Can you work these out from the model? Positions are in its coordinate system, mm. Face numbers are marked on the shaded views. Give positions to 0.01 mm unless a question says otherwise; leave off trailing zeros. Write each loop counter-clockwise with the first axis right and the second up, starting at its lowest first coordinate (ties: lowest second). Pieces come first, ordered by that corner, then holes. Notation, with made-up numbers: (69.25, 82) -> (81.25, 82) arc R14 cw to (81.25, 89) -> close; hole circle Ø5 at (55, 82.25). An arc over 180 degrees is marked (long way). Answer as CSV lines item,"result". Start each with the question number.
1. If we section it at A-A on y = 14: Count the separate pieces of the cut face and the enclosed holes in it, plus the area to 3 significant figures.
2. I'm going to push flat-ended pins straight in: P1, Ø3, axis at x = 28.5, z = -5.5, coming from the -Y side; P2, Ø2, axis at x = 42.5, y = 13.5, coming from the -Z side; P3, Ø3, axis at y = 13.5, z = -19.5, coming from the +X side; P4, Ø3, axis at x = 72.5, y = 14.5, coming from the +Z side. Where does each tip first touch, or does it pass through?
3. If we mould it in two halves opening along X, with no side actions, what happens to the marked faces 1 and 2? For each: pulls with the +X half, pulls with the -X half, needs draft (parallel to the pull), parting line crosses it, or undercut.
4. I need wall thicknesses on line 1 (Z direction, x = 28.5, y = 3.5); line 2 (Z direction, x = 28.5, y = 2.1) (3 decimals); line 3 (X direction, y = 3.4, z = -5.5). Which ranges of each line are inside material? Lowest first, please. Write a range as [from, to].
5. If we section it at B-B on x = 168.5: Write out the boundary of the cut face in (y, z), plus the area to 3 significant figures.
```python
from build123d import *

# Parameters (mm, degrees)
SKETCH1_W                = 240
SKETCH1_H                = 35
SKETCH1_W_2              = 12.7
SKETCH1_H_2              = 12.7
BOSS_EXTRUDE1_DEPTH      = 4
SKETCH2_W                = 12.7
SKETCH2_H                = 12.7
BOSS_EXTRUDE2_DEPTH      = 13
BOSS_EXTRUDE2_DEPTH_BACK = 4
CHAMFER1_SIZE            = 0.2
CHAMFER1_SIZE2           = 8
SKETCH3_R                = 1.725
CUT_EXTRUDE1_DEPTH       = 5
SKETCH4_R                = 3
CUT_EXTRUDE2_DEPTH       = 1
FILLET1_R                = 1


with BuildPart() as part:
    # Sketch1 → Boss-Extrude1 (new body)
    with BuildSketch(Plane(origin=(0, 0, 0), x_dir=(1, 0, 0), z_dir=(0, 1, 0))):
        with Locations((120, 17.5)):
            Rectangle(SKETCH1_W, SKETCH1_H)
        with Locations((13.25, 17.5)):
            Rectangle(SKETCH1_W_2, SKETCH1_H_2, mode=Mode.SUBTRACT)
        with Locations((43.75, 17.5)):
            Rectangle(SKETCH1_W_2, SKETCH1_H_2, mode=Mode.SUBTRACT)
        with Locations((74.25, 17.5)):
            Rectangle(SKETCH1_W_2, SKETCH1_H_2, mode=Mode.SUBTRACT)
        with Locations((104.75, 17.5)):
            Rectangle(SKETCH1_W_2, SKETCH1_H_2, mode=Mode.SUBTRACT)
        with Locations((135.25, 17.5)):
            Rectangle(SKETCH1_W_2, SKETCH1_H_2, mode=Mode.SUBTRACT)
        with Locations((165.75, 17.5)):
            Rectangle(SKETCH1_W_2, SKETCH1_H_2, mode=Mode.SUBTRACT)
        with Locations((196.25, 17.5)):
            Rectangle(SKETCH1_W_2, SKETCH1_H_2, mode=Mode.SUBTRACT)
        with Locations((226.75, 17.5)):
            Rectangle(SKETCH1_W_2, SKETCH1_H_2, mode=Mode.SUBTRACT)
    extrude(amount=BOSS_EXTRUDE1_DEPTH)

    # Sketch2 → Boss-Extrude2 (add, two sides)
    with BuildSketch(Plane(origin=(0, 4, 0), x_dir=(1, 0, 0), z_dir=(0, 1, 0))) as boss_extrude2_sk:
        with Locations((13.25, 17.5)):
            Rectangle(SKETCH2_W, SKETCH2_H)
        with Locations((43.75, 17.5)):
            Rectangle(SKETCH2_W, SKETCH2_H)
        with Locations((74.25, 17.5)):
            Rectangle(SKETCH2_W, SKETCH2_H)
        with Locations((104.75, 17.5)):
            Rectangle(SKETCH2_W, SKETCH2_H)
        with Locations((135.25, 17.5)):
            Rectangle(SKETCH2_W, SKETCH2_H)
        with Locations((165.75, 17.5)):
            Rectangle(SKETCH2_W, SKETCH2_H)
        with Locations((196.25, 17.5)):
            Rectangle(SKETCH2_W, SKETCH2_H)
        with Locations((226.75, 17.5)):
            Rectangle(SKETCH2_W, SKETCH2_H)
    extrude(amount=BOSS_EXTRUDE2_DEPTH)
    extrude(boss_extrude2_sk.sketch, amount=-BOSS_EXTRUDE2_DEPTH_BACK)

    # Chamfer1
    chamfer1_edges = [part.edges().sort_by_distance(p)[0] for p in [
        (189.9, 4, -17.5),
        (196.25, 4, -11.15),
        (202.6, 4, -17.5),
        (196.25, 4, -23.85),
        (6.9, 4, -17.5),
        (13.25, 4, -11.15),
        (19.6, 4, -17.5),
        (13.25, 4, -23.85),
        (67.9, 4, -17.5),
        (74.25, 4, -11.15),
        (80.6, 4, -17.5),
        (74.25, 4, -23.85),
        (37.4, 4, -17.5),
        (43.75, 4, -11.15),
        (50.1, 4, -17.5),
        (43.75, 4, -23.85),
        (98.4, 4, -17.5),
        (104.75, 4, -11.15),
        (111.1, 4, -17.5),
        (104.75, 4, -23.85),
        (128.9, 4, -17.5),
        (135.25, 4, -11.15),
        (141.6, 4, -17.5),
        (135.25, 4, -23.85),
        (159.4, 4, -17.5),
        (165.75, 4, -11.15),
        (172.1, 4, -17.5),
        (165.75, 4, -23.85),
        (220.4, 4, -17.5),
        (226.75, 4, -11.15),
        (233.1, 4, -17.5),
        (226.75, 4, -23.85),
    ]]
    chamfer1_side = [part.faces().sort_by_distance(p)[0] for p in [
        (120, 4, -17.5),
    ]]
    chamfer(chamfer1_edges, length=CHAMFER1_SIZE, length2=CHAMFER1_SIZE2, reference=chamfer1_side[0])

    # Sketch3 → Cut-Extrude1 (cut, through all)
    with BuildSketch(Plane(origin=(0, 4, 0), x_dir=(1, 0, 0), z_dir=(0, 1, 0))):
        with Locations((28.5, 5.5)):
            Circle(SKETCH3_R)
        with Locations((28.5, 29.5)):
            Circle(SKETCH3_R)
        with Locations((211.6, 29.5)):
            Circle(SKETCH3_R)
        with Locations((211.6, 5.5)):
            Circle(SKETCH3_R)
    extrude(amount=-CUT_EXTRUDE1_DEPTH, mode=Mode.SUBTRACT)

    # Sketch4 → Cut-Extrude2 (cut)
    with BuildSketch(Plane(origin=(0, 4, 0), x_dir=(1, 0, 0), z_dir=(0, 1, 0))):
        with Locations((28.5, 29.5)):
            Circle(SKETCH4_R)
        with Locations((28.5, 5.5)):
            Circle(SKETCH4_R)
        with Locations((211.6, 5.5)):
            Circle(SKETCH4_R)
        with Locations((211.6, 29.5)):
            Circle(SKETCH4_R)
    extrude(amount=-CUT_EXTRUDE2_DEPTH, mode=Mode.SUBTRACT)

    # Fillet1
    fillet1_edges = [part.edges().sort_by_distance(p)[0] for p in [
        (6.9, 17, -17.5),
        (13.25, 17, -11.15),
        (19.6, 17, -17.5),
        (13.25, 17, -23.85),
        (37.4, 17, -17.5),
        (43.75, 17, -11.15),
        (50.1, 17, -17.5),
        (43.75, 17, -23.85),
        (67.9, 17, -17.5),
        (74.25, 17, -11.15),
        (80.6, 17, -17.5),
        (74.25, 17, -23.85),
        (98.4, 17, -17.5),
        (104.75, 17, -11.15),
        (111.1, 17, -17.5),
        (104.75, 17, -23.85),
        (128.9, 17, -17.5),
        (135.25, 17, -11.15),
        (141.6, 17, -17.5),
        (135.25, 17, -23.85),
        (159.4, 17, -17.5),
        (165.75, 17, -11.15),
        (172.1, 17, -17.5),
        (165.75, 17, -23.85),
        (189.9, 17, -17.5),
        (196.25, 17, -11.15),
        (202.6, 17, -17.5),
        (196.25, 17, -23.85),
        (220.4, 17, -17.5),
        (226.75, 17, -11.15),
        (233.1, 17, -17.5),
        (226.75, 17, -23.85),
    ]]
    fillet(fillet1_edges, radius=FILLET1_R)


solid = part.part
```
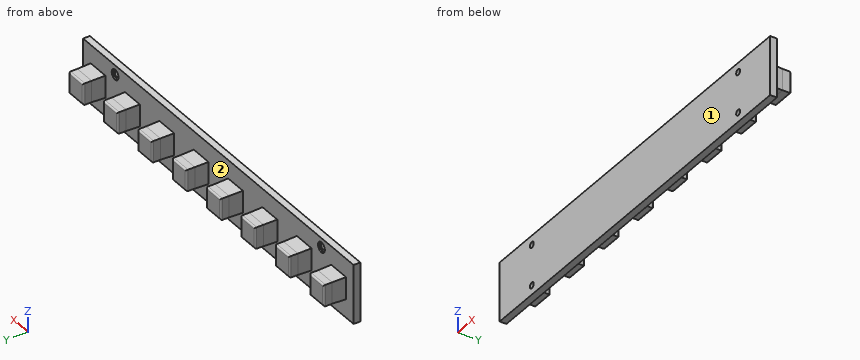
Computed values:
1,separate pieces,"8"
1,enclosed holes,"0"
1,area,"1,290 mm2"
2,P1,"passes through"
2,P2,"stops at z = -23.85"
2,P3,"stops at x = 233.1"
2,P4,"stops at z = -11.15"
3,face 1,"needs draft"
3,face 2,"undercut"
4,line 1,"z = [-35, -32.5], [-26.5, -8.5], [-2.5, 0]"
4,line 2,"z = [-35, -31.225], [-27.775, -7.225], [-3.775, 0]"
4,line 3,"x = [0, 25.5], [31.5, 208.6], [214.6, 240]"
5,outline,"(0, -35) -> (4, -35) -> (4, -24.05) -> (12, -23.85) -> (16, -23.85) arc R1 ccw to (17, -22.85) -> (17, -12.15) arc R1 ccw to (16, -11.15) -> (12, -11.15) -> (4, -10.95) -> (4, 0) -> (0, 0) -> close"
5,area,"306 mm2"
